Read the model definition and answer for the solid it produces. Units are mm, in the model's axes. A direction names the side the tool comes from. Coordinates: 2 decimals unless noted, no trailing zeros. Order: outer loops, then holes, each group sorted by start corner. A loop starts at its lowest first (then second) coordinate and runs counter-clockwise, first axis right, second up. Notation, with made-up numbers: (45, -21) -> (69, -21) arc R13 ccw to (69, 4) -> close; hole circle Ø7 at (60, 81). An arc over 180 degrees is marked (long way). Answer as a JSON object with one key per item and string values. Group by question number.
1) Section C-C on x = 10.5 is taken. Determine the outline of the cut face in (y, z).
2) Section B-B on z = -30 is taken. Determine the outline of the cut face in (x, y).
3) Section A-A on z = -9 is taken. Determine the outline of the cut face in (x, y), and give its area (3 significant figures).
4) Consider L1, parallel to Y at x = 7, z = -10.5; L2, parallel to X at y = 8.75, z = -3; L3, parallel to X at y = 1.25, z = -24.5. Determine where each line is inside the solid, lowest interval first.
5) A tool of negligible diameter and unlimited length cuts with its end or side. For faces 1 (the flat face through (11, 7, -16)), 2 (the flat face through (6, 0, -16)), from which of +Z, -Z, +X, -X, +Y, -Y can it reach the whole face along a straight path? Write none if from no direction.
6) Section D-D on y = 6.75 is taken. Determine the outline of the cut face in (x, z).
7) Given pin 1 (5.5 mm diameter, centred on y = 7, z = -11.5, fed in from -X), flat-ended and moving along its own axis, determine where the tip first touches the part or whether it passes through.
from build123d import *

# Parameters (mm, degrees)
SKETCH1_W           = 11
SKETCH1_H           = 32
BOSS_EXTRUDE1_DEPTH = 2
SKETCH4_W           = 32
SKETCH4_H           = 2
BOSS_EXTRUDE2_DEPTH = 2
SKETCH5_W           = 2
SKETCH5_H           = 32
BOSS_EXTRUDE3_DEPTH = 11
CUT_EXTRUDE6_DEPTH  = 37.249137921


with BuildPart() as part:
    # Sketch1 → Boss-Extrude1 (new body)
    with BuildSketch(Plane(origin=(0, 0, 0), x_dir=(1, 0, 0), z_dir=(0, 1, 0))):
        with Locations((5.5, 16)):
            Rectangle(SKETCH1_W, SKETCH1_H)
    extrude(amount=BOSS_EXTRUDE1_DEPTH)

    # Sketch4 → Boss-Extrude2 (add)
    with BuildSketch(Plane(origin=(11, 0, 0), x_dir=(0, 0, -1), z_dir=(1, 0, 0))):
        with Locations((16, 1)):
            Rectangle(SKETCH4_W, SKETCH4_H)
    extrude(amount=BOSS_EXTRUDE2_DEPTH)

    # Sketch5 → Boss-Extrude3 (add)
    with BuildSketch(Plane(origin=(0, 2, 0), x_dir=(1, 0, 0), z_dir=(0, 1, 0))):
        with Locations((12, 16)):
            Rectangle(SKETCH5_W, SKETCH5_H)
    extrude(amount=BOSS_EXTRUDE3_DEPTH)

    # Sketch6 → Cut-Extrude6 (cut, through all)
    with BuildSketch(Plane(origin=(0, 2, 0), x_dir=(1, 0, 0), z_dir=(0, 1, 0))):
        with BuildLine():
            ThreePointArc((7.5, 8), (6.914213562, 9.414213562), (5.5, 10))
            Line((5.5, 10), (5.5, 6))
            ThreePointArc((5.5, 6), (6.914213562, 6.585786438), (7.5, 8))
        make_face()
        with BuildLine():
            Line((5.5, 6), (5.5, 10))
            ThreePointArc((5.5, 10), (3.5, 8), (5.5, 6))
        make_face()
        with BuildLine():
            ThreePointArc((5.5, 26), (3.5, 24), (5.5, 22))
            Line((5.5, 22), (5.5, 26))
        make_face()
        with BuildLine():
            Line((5.5, 26), (5.5, 22))
            ThreePointArc((5.5, 22), (6.914213562, 22.585786438), (7.5, 24))
            ThreePointArc((7.5, 24), (6.914213562, 25.414213562), (5.5, 26))
        make_face()
    extrude(amount=-CUT_EXTRUDE6_DEPTH, mode=Mode.SUBTRACT)


solid = part.part
Worked answers:
{
 "1": {"outline": "(0, -32) -> (2, -32) -> (2, 0) -> (0, 0) -> close"},
 "2": {"outline": "(0, 0) -> (13, 0) -> (13, 13) -> (11, 13) -> (11, 2) -> (0, 2) -> close"},
 "3": {"outline": "(0, 0) -> (3.77, 0) -> (3.77, 2) -> (0, 2) -> close; (7.23, 0) -> (13, 0) -> (13, 13) -> (11, 13) -> (11, 2) -> (7.23, 2) -> close", "area": "41.1 mm²"},
 "4": {"L1": "y = 0 to 2", "L2": "x = 11 to 13", "L3": "x = 0 to 3.56, 7.44 to 13"},
 "5": {"face 1": "+Z, -Z, -X, +Y", "face 2": "+Z, -Z, +X, -X, -Y"},
 "6": {"outline": "(11, -32) -> (13, -32) -> (13, 0) -> (11, 0) -> close"},
 "7": {"pin 1": "stops at x = 11"}
}
